Can you work these out from the model? Positions are in its coordinate system, mm. A direction names the side the tool comes from. Round coordinates to 2 decimals unless told otherwise and drop trailing zeros. Loops run counter-clockwise (first coordinate to the right, second up) from the corner with the lowest first, then second, coordinate; pieces in that order, holes last. Notation, with made-up numbers: (43, 80.5) -> (47, 80.5) arc R26 ccw to (47, 116.5) -> close; hole circle Ø1 at (13.25, 41.25). An arc over 180 degrees is marked (long way). Write item = value, one per line.
from build123d import *

# Parameters (mm, degrees)
SKETCH1_W                   = 42
SKETCH1_H                   = 40.2
BOSS_EXTRUDE1_DEPTH         = 5
SKETCH2_W                   = 31.6
SKETCH2_H                   = 12.6
CUT_EXTRUDE1_DEPTH          = 3
SKETCH3_W                   = 25.6
SKETCH3_H                   = 7.6
CUT_EXTRUDE2_DEPTH          = 3
CUT_EXTRUDE3_DEPTH          = 5
FILLET1_R                   = 2
SKETCH9_W                   = 41
SKETCH9_H                   = 2
BOSS_EXTRUDE3_DEPTH         = 10
FILLET2_R                   = 1
TAP_DRILL_FOR_M3_TAP1_D     = 2.5
TAP_DRILL_FOR_M3_TAP1_DEPTH = 2
TAP_DRILL_FOR_M3_TAP1_TIP   = 0.751075774
FILLET3_R                   = 1


with BuildPart() as part:
    # Sketch1 → Boss-Extrude1 (new body)
    with BuildSketch(Plane.XY):
        with Locations((-0.5, 2.1)):
            Rectangle(SKETCH1_W, SKETCH1_H)
    extrude(amount=BOSS_EXTRUDE1_DEPTH)

    # Sketch2 → Cut-Extrude1 (cut)
    with BuildSketch(Plane.XY.offset(5)):
        with Locations((-1, 10.7)):
            Rectangle(SKETCH2_W, SKETCH2_H)
        with Locations((-1, -6.5)):
            Rectangle(SKETCH2_W, SKETCH2_H)
    extrude(amount=-CUT_EXTRUDE1_DEPTH, mode=Mode.SUBTRACT)

    # Sketch3 → Cut-Extrude2 (cut)
    with BuildSketch(Plane.XY.offset(2)):
        with Locations((-1, 10.7)):
            Rectangle(SKETCH3_W, SKETCH3_H)
        with Locations((-1, -6.5)):
            Rectangle(SKETCH3_W, SKETCH3_H)
    extrude(amount=-CUT_EXTRUDE2_DEPTH, mode=Mode.SUBTRACT)

    # Sketch4 → Cut-Extrude3 (cut)
    with BuildSketch(Plane(origin=(0, 0, 0), x_dir=(-1, 0, 0), z_dir=(0, 0, -1))):
        Polygon((-15.288574128, 22.2), (-20.5, 22.2), (-20.5, 16.307906388), (-20.5, -16.83473783), (-20.5, -18), (-15.288574128, -18), (16.313805872, -18), (21.5, -18), (21.5, -16.83473783), (21.5, -16.1), (-19.5, -16.1), (-19.5, 18.5), (21.5, 18.5), (21.5, 22.2), (16.313805872, 22.2), align=None)
    extrude(amount=-CUT_EXTRUDE3_DEPTH, mode=Mode.SUBTRACT)

    # Fillet1
    fillet1_edges = [part.edges().sort_by_distance(p)[0] for p in [
        (-13.8, 6.9, 1),
        (-13.8, 14.5, 1),
        (11.8, 14.5, 1),
        (11.8, 6.9, 1),
        (-13.8, -10.3, 1),
        (-13.8, -2.7, 1),
        (11.8, -2.7, 1),
        (11.8, -10.3, 1),
        (19.5, 18.5, 2.5),
        (-21.5, 18.5, 2.5),
    ]]
    fillet(fillet1_edges, radius=FILLET1_R)

    # Sketch9 → Boss-Extrude3 (add)
    with BuildSketch(Plane.XY.offset(5)):
        with Locations((-1, -17.1)):
            Rectangle(SKETCH9_W, SKETCH9_H)
    extrude(amount=-BOSS_EXTRUDE3_DEPTH)

    # Fillet2
    fillet2_edges = [part.edges().sort_by_distance(p)[0] for p in [
        (-1, -18.1, 5),
    ]]
    fillet(fillet2_edges, radius=FILLET2_R)

    # Tap Drill for M3 Tap1
    with Locations(Plane(origin=(0, -16.1, 0), x_dir=(1, 0, 0), z_dir=(0, 1, 0))):
        with Locations((14, 2.87743455), (4, 2.87743455), (-6, 2.87743455), (-16, 2.87743455)):
            Hole(TAP_DRILL_FOR_M3_TAP1_D / 2, depth=TAP_DRILL_FOR_M3_TAP1_DEPTH)
            with Locations((0, 0, -(TAP_DRILL_FOR_M3_TAP1_DEPTH + TAP_DRILL_FOR_M3_TAP1_TIP / 2))):  # 118° drill point
                Cone(0, TAP_DRILL_FOR_M3_TAP1_D / 2, TAP_DRILL_FOR_M3_TAP1_TIP, mode=Mode.SUBTRACT)

    # Fillet3
    fillet3_edges = [part.edges().sort_by_distance(p)[0] for p in [
        (-21.5, -17.1, -5),
        (19.5, -17.1, -5),
    ]]
    fillet(fillet3_edges, radius=FILLET3_R)


solid = part.part
1. Suppose I cut it at C-C, the plane y = 12. List the corners of the cut face in (x, z) for me, and give its area (3 significant figures).
Entries:
outline = (-21.5, 0) -> (-13.8, 0) -> (-13.8, 2) -> (-16.8, 2) -> (-16.8, 5) -> (-21.5, 5) -> close; (11.8, 0) -> (19.5, 0) -> (19.5, 5) -> (14.8, 5) -> (14.8, 2) -> (11.8, 2) -> close
area = 59.0 mm²
2. Suppose I cut it at B-B, the plane z = 2.75. List the corners of the cut face in (x, y) for me.
Entries:
outline = (-21.5, -18.1) -> (19.5, -18.1) -> (19.5, 16.5) arc R2 ccw to (17.5, 18.5) -> (-19.5, 18.5) arc R2 ccw to (-21.5, 16.5) -> close; hole (-16.8, -12.8) -> (14.8, -12.8) -> (14.8, -0.2) -> (-16.8, -0.2) -> close; hole (-16.8, 4.4) -> (14.8, 4.4) -> (14.8, 17) -> (-16.8, 17) -> close
3. Suppose I cut it at A-A, the plane x = -6. List the corners of the cut face in (y, z) for me.
Entries:
outline = (-18.1, -5) -> (-16.1, -5) -> (-16.1, -4.13) -> (-18.1, -4.13) -> close; (-18.1, -1.63) -> (-16.1, -1.63) -> (-16.1, 0) -> (-10.3, 0) -> (-10.3, 2) -> (-12.8, 2) -> (-12.8, 5) -> (-17.1, 5) arc R1 ccw to (-18.1, 4) -> close; (-2.7, 0) -> (6.9, 0) -> (6.9, 2) -> (4.4, 2) -> (4.4, 5) -> (-0.2, 5) -> (-0.2, 2) -> (-2.7, 2) -> close; (14.5, 0) -> (18.5, 0) -> (18.5, 5) -> (17, 5) -> (17, 2) -> (14.5, 2) -> close
4. I'm going to push flat-ended pins straight in: pin 1 (5 mm diameter, centred on x = -6.5, y = 1, fed in from -Z); pin 2 (3 mm diameter, centred on x = -16, z = -2.88, fed in from +Y). Where does each tip first touch, or does it pass through?
Entries:
pin_1 = 0
pin_2 = -16.1
5. I need wall thicknesses on line 1 (Y direction, x = -13, z = 4); line 2 (Y direction, x = 6, z = 1.25); line 3 (Z direction, x = -16, y = -17). Which ranges of each line are inside material? Lowest first, please. Write a range as [from, to].
Entries:
line_1 = [-18.1, -12.8], [-0.2, 4.4], [17, 18.5]
line_2 = [-18.1, -10.3], [-2.7, 6.9], [14.5, 18.5]
line_3 = [-5, -4.13], [-1.63, 5]
6. Suppose I cut it at D-D, the plane x = 1. List the corners of the cut face in (y, z) for me, and give its area (3 significant figures).
Entries:
outline = (-18.1, -5) -> (-16.1, -5) -> (-16.1, 0) -> (-10.3, 0) -> (-10.3, 2) -> (-12.8, 2) -> (-12.8, 5) -> (-17.1, 5) arc R1 ccw to (-18.1, 4) -> close; (-2.7, 0) -> (6.9, 0) -> (6.9, 2) -> (4.4, 2) -> (4.4, 5) -> (-0.2, 5) -> (-0.2, 2) -> (-2.7, 2) -> close; (14.5, 0) -> (18.5, 0) -> (18.5, 5) -> (17, 5) -> (17, 2) -> (14.5, 2) -> close
area = 86.8 mm²
7. For faces 1 (the cylindrical face through (-20.93, 17.9, 2.54)), 2 (the flat face through (14.8, 11, 4)), 3 (the flat face through (-1, 6.9, 1)), which set-ups out of +Z, -Z, +X, -X, +Y, -Y let a thin tool reach every point of the face, with its end or its side?
Entries:
face_1 = +Z, -Z, -X, +Y
face_2 = +Z
face_3 = +Z, -Z
8. We'd pull the mould along Z, two halves only. Please class faces 4 (the cylindrical face through (-17.155, -17.114, -2.399)), 5 (the flat face through (-1, -17, -5)), 6 (the flat face through (-1, -12.8, 4)), 7 (the cylindrical face through (15.25, -17.11, -2.93)): released by +Z, released by -Z, zero draft, split by the parting line, or undercut.
Entries:
face_4 = undercut
face_5 = released by -Z
face_6 = zero draft
face_7 = undercut
